CAD build for the part. Positions are in the model's coordinates, mm. Face numbers are marked on the shaded views. A direction names the side the tool comes from. Coordinates: 2 decimals unless noted, no trailing zeros. Write each loop counter-clockwise with the first axis right and the second up, starting at its lowest first coordinate (ties: lowest second). Pieces come first, ordered by that corner, then holes. Notation, with made-up numbers: (22.25, -6) - (43.25, -6) arc R22 cw to (43.25, 0) - close; hole circle Ø2 at (11, 65.25). An arc over 180 degrees is marked (long way). Answer in a Markdown table with one row per item. Add a question column.
Q1. Band-saw the part on C-C (z = 18). List the corners of the cut face in (x, y).
Q2. Band-saw the part on A-A (x = 12.5). List the corners of the cut face in (y, z).
Q3. Band-saw the part on D-D (x = 18.5). List the corners of the cut face in (y, z).
Q4. Band-saw the part on B-B (y = 14.25). List the corners of the cut face in (x, z).
Q5. Pin check, flat tips, straight feed: pin 1 (5.5 mm diameter, centred on x = 22.5, z = 20.5, fed in from -Y); pin 2 (6.5 mm diameter, centred on x = 11, y = 9, fed in from +Z). Stop position of each tip, or through.
Q6. Two-plate mould, pull along X, no slides. Class the marked faces 1, 2, 3 and 4: +X half, -X half, draft (parallel to the pull), parting line (faces both ways), or undercut.
Q7. 3-axis set-ups, long thin cutter, end or side, ignore diameter. For the marked faces 5, 6 and 7: which of +Z, -Z, +X, -X, +Y, -Y reach the whole face in a straight line?
Q8. Drill centre lines: line 1 along X through (y, z) = (18.75, 30); line 2 along Y through (x, z) = (22, 16.5); line 3 along Z through (x, y) = (20, 8). Where is each one in solid material? Low to high. Write a range as from..to.
```python
from build123d import *

# Parameters (mm, degrees)
F1_DEPTH = 38.1
F2_W     = 11.3489339128
F2_H     = 7.6335099638
F3_DEPTH = 6.35
F4_DEPTH = 12.7


with BuildPart() as f1:
    # F0 (on Right) → F1 (new body)
    with BuildSketch(Plane.YZ):
        Polygon((0, 12.7), (0, 0), (25.4, 0), (25.4, 31.75), (12.7, 31.75), (12.7, 12.7), align=None)
    extrude(amount=F1_DEPTH)

    # F2 (on face) → F3 (cut)
    with BuildSketch(Plane.XZ.offset(-12.7)):
        with Locations((19.8606378399, 27.9332450181)):
            Rectangle(F2_W, F2_H)
    extrude(amount=-F3_DEPTH, mode=Mode.SUBTRACT)

    # F4 (cut): a face of the model
    f4_faces = [f1.faces().sort_by_distance(p)[0] for p in [
        (19.8606378399, 19.05, 27.9332450181),
    ]]
    extrude(f4_faces, amount=-F4_DEPTH, mode=Mode.SUBTRACT)


solid = f1.part
```
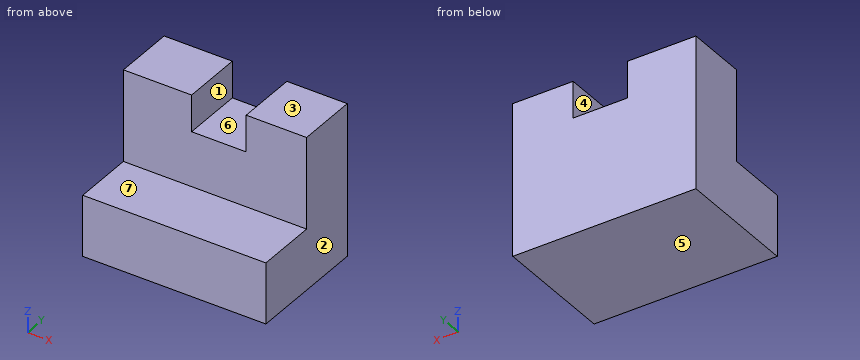
Checked values:
| question | item | result |
|---|---|---|
| 1 | outline | (0, 12.7) - (38.1, 12.7) - (38.1, 25.4) - (0, 25.4) - close |
| 2 | outline | (0, 0) - (25.4, 0) - (25.4, 31.75) - (12.7, 31.75) - (12.7, 12.7) - (0, 12.7) - close |
| 3 | outline | (0, 0) - (25.4, 0) - (25.4, 24.12) - (12.7, 24.12) - (12.7, 12.7) - (0, 12.7) - close |
| 4 | outline | (0, 0) - (38.1, 0) - (38.1, 31.75) - (25.54, 31.75) - (25.54, 24.12) - (14.19, 24.12) - (14.19, 31.75) - (0, 31.75) - close |
| 5 | pin 1 | stops at y = 12.7 |
| 5 | pin 2 | stops at z = 12.7 |
| 6 | face 1 | undercut |
| 6 | face 2 | +X half |
| 6 | face 3 | draft |
| 6 | face 4 | undercut |
| 7 | face 5 | -Z, +X, -X, +Y, -Y |
| 7 | face 6 | +Z, +Y, -Y |
| 7 | face 7 | +Z, +X, -X, -Y |
| 8 | line 1 | x = 0..14.19, 25.54..38.1 |
| 8 | line 2 | y = 12.7..25.4 |
| 8 | line 3 | z = 0..12.7 |
